```python
from build123d import *

# Parameters (mm, degrees)
F0_W     = 101.6
F0_H     = 55.626
F1_DEPTH = 50
F2_R     = 5
F3_T     = -2.5


with BuildPart() as f1:
    # F0 (on Front) → F1 (new body)
    with BuildSketch(Plane.XZ):
        Rectangle(F0_W, F0_H)
    extrude(amount=F1_DEPTH)

    # F2
    f2_edges = [f1.edges().sort_by_distance(p)[0] for p in [
        (-50.8, -50, 0),
        (50.8, -50, 0),
        (50.8, 0, 0),
        (-50.8, 0, 0),
    ]]
    fillet(f2_edges, radius=F2_R)

    # F3
    f3_openings = [f1.faces().sort_by_distance(p)[0] for p in [
        (0, -25, 27.813),
        (0, -25, -27.813),
    ]]
    offset(amount=F3_T, openings=f3_openings)


solid = f1.part
```
Design review of the part built by this model. Coordinates are the model's own, in mm. A direction names the side the tool comes from. Give positions to 0.01 mm unless a question says otherwise; leave off trailing zeros. Order: outer loops, then holes, each group sorted by start corner. A loop starts at its lowest first (then second) coordinate and runs counter-clockwise, first axis right, second up. Notation, with made-up numbers: (34.25, 20.25) - (38.25, 20.25) arc R16 cw to (38.25, 27.25) - close; hole circle Ø10 at (84.25, 37.5). An arc over 180 degrees is marked (long way). Use a Markdown table: item, result. Add a question column.
(1) Add section C-C on z = -4.5. Give the boundary of the cut face in (x, y).
(2) Wall thickness on probe 1 along X at (y, z) = (-37, -5); probe 2 along Y at (x, z) = (-30.5, -8.5); probe 3 along X at (y, z) = (-48, -17): over which ranges is each line inside the solid? List them lowest first. Write a range as [from, to].
(3) Add section A-A on y = -28.5. Give the boundary of the cut face in (x, z), then the cut area to 3 significant figures.
(4) Mouldability with a two-part tool opening along X and no side actions: class faces 3 (the face through (50.8, -25, 0)), 4 (the face through (-48.3, -25, 0)), 5 (the face through (0, -49, 27.813)) as +X half, -X half, draft (parallel to the pull), parting line (faces both ways), or undercut.
(5) Clearance check with a flat-ended pin moving along its axis: P1, Ø6, axis at x = 29.5, y = -45, coming from the -Z side. State where the tip first meets the part, or that it passes through.
(6) Add section B-B on x = -38. Give the boundary of the cut face in (y, z).
(7) Machinability: for faces 1 (the face through (0, -49, -27.813)), 2 (the face through (47.587, -46.748, 0.389)), which of the approach directions +Z, -Z, +X, -X, +Y, -Y give a long, thin tool a straight path to every point of the face, cutting with its end or side? Answer none if there is none.
Report:
| question | item | result |
|---|---|---|
| 1 | outline | (-50.8, -45) arc R5 ccw to (-45.8, -50) - (45.8, -50) arc R5 ccw to (50.8, -45) - (50.8, -5) arc R5 ccw to (45.8, 0) - (-45.8, 0) arc R5 ccw to (-50.8, -5) - close; hole (-48.3, -45) arc R2.5 ccw to (-45.8, -47.5) - (45.8, -47.5) arc R2.5 ccw to (48.3, -45) - (48.3, -5) arc R2.5 ccw to (45.8, -2.5) - (-45.8, -2.5) arc R2.5 ccw to (-48.3, -5) - close |
| 2 | probe 1 | x = [-50.8, -48.3], [48.3, 50.8] |
| 2 | probe 2 | y = [-50, -47.5], [-2.5, 0] |
| 2 | probe 3 | x = [-49.8, 49.8] |
| 3 | outline | (-50.8, -27.81) - (-48.3, -27.81) - (-48.3, 27.81) - (-50.8, 27.81) - close; (48.3, -27.81) - (50.8, -27.81) - (50.8, 27.81) - (48.3, 27.81) - close |
| 3 | area | 278 mm² |
| 4 | face 3 | +X half |
| 4 | face 4 | undercut |
| 4 | face 5 | draft |
| 5 | P1 | stops at z = -27.81 |
| 6 | outline | (-50, -27.81) - (-47.5, -27.81) - (-47.5, 27.81) - (-50, 27.81) - close; (-2.5, -27.81) - (0, -27.81) - (0, 27.81) - (-2.5, 27.81) - close |
| 7 | face 1 | -Z, +X, -X, +Y, -Y |
| 7 | face 2 | +Z, -Z |
